Geometry: final body of the model. Coordinates: model frame, mm. A direction names the side the tool comes from. Round coordinates to 2 decimals unless told otherwise and drop trailing zeros. Order: outer loops, then holes, each group sorted by start corner. A loop starts at its lowest first (then second) coordinate and runs counter-clockwise, first axis right, second up. Notation, with made-up numbers: M 65,24.5 L 81,24.5 A17 cw 81,53.5 Z; hole C 30,-39.75 d1. An arc over 180 degrees is marked long. Put each result on its own line as item: value. Start each with the question number.
1) Access query for faces 5 (the cylindrical face through (-12.347, 2.37, -0.275)), 6 (the flat face through (-8, 0, 0)). Directions: +Z, -Z, +X, -X, +Y, -Y. A direction counts if a zero-diameter tool reaches every point of the face in a straight line with its end or side. Return the directions, or none.
2) Draft query along Z for faces 1 (the flat face through (-6, 3.175, 0)), 2 (the flat face through (-6, 2, -1.588)), 3 (the flat face through (-6, 2, 1.588)), 4 (the flat face through (-11, 1.588, 0)). Return one class per face: pulls with the +Z half, pulls with the -Z half, needs draft (parallel to the pull), parting line crosses it, or undercut.
3) Section C-C, the plane y = 2.2. Return loops of the section in (x, z) (1 decimal), then the cut area to 3 significant figures.
4) First-contact query: P1, Ø0.8, axis at x = -11, z = 0, coming from the +Y side; P2, Ø1, axis at x = -11, z = 0, coming from the -Y side. Flat tips, straight axial feed; report the tip coordinate or a pass-through.
5) Section B-B, the plane x = -1.25. Return loops of the section in (y, z) (1 decimal).
6) Material intervals for probe 1 along X at (y, z) = (2.3, 0); probe 2 along X at (y, z) = (1.85, -0.3); probe 3 along X at (y, z) = (1.1, -0.05), sorted ascending. Write a range as [from, to].
from build123d import *

# Parameters (mm, degrees)
BOSS_EXTRUDE2_DEPTH = 3.175
SKETCH1_6_W         = 3.175
SKETCH1_6_H         = 3.175
SKETCH1_6_R         = 1.27
BOSS_EXTRUDE6_DEPTH = 3.175
SKETCH1_8_R         = 1.27
BOSS_EXTRUDE7_DEPTH = 1.5875


with BuildPart() as part:
    # Sketch1 → Boss-Extrude2 (new body)
    with BuildSketch(Plane(origin=(0, 0, 0), x_dir=(1, 0, 0), z_dir=(0, 1, 0))):
        with BuildLine():
            Line((-2.749630657, 1.5875), (-9.525, 1.5875))
            Line((-9.525, 1.5875), (-9.525, -1.5875))
            Line((-9.525, -1.5875), (-2.749630657, -1.5875))
            Line((-2.749630657, -1.5875), (0, -1.5875))
            ThreePointArc((0, -1.5875), (-1.5875, 0), (0, 1.5875))
            Line((0, 1.5875), (-2.749630657, 1.5875))
        make_face()
    extrude(amount=BOSS_EXTRUDE2_DEPTH)

    # Sketch1<6> → Boss-Extrude6 (add)
    with BuildSketch(Plane(origin=(0, 0, 0), x_dir=(1, 0, 0), z_dir=(0, 1, 0))):
        with Locations((-11.1125, 0)):
            Rectangle(SKETCH1_6_W, SKETCH1_6_H)
        with Locations(Location((-11.107619253, 0, 0), (0, 0, 270))):
            Circle(SKETCH1_6_R, mode=Mode.SUBTRACT)
    extrude(amount=BOSS_EXTRUDE6_DEPTH)

    # Sketch1<8> → Boss-Extrude7 (add)
    with BuildSketch(Plane(origin=(0, 0, 0), x_dir=(1, 0, 0), z_dir=(0, 1, 0))):
        with Locations(Location((-11.107619253, 0, 0), (0, 0, 270))):
            Circle(SKETCH1_8_R)
    extrude(amount=BOSS_EXTRUDE7_DEPTH)


solid = part.part
Result sheet:
1. face 5: +Y
1. face 6: +Z, -Z, +X, -X, -Y
2. face 1: needs draft
2. face 2: pulls with the -Z half
2. face 3: pulls with the +Z half
2. face 4: undercut
3. outline: M -12.7,-1.6 L 0,-1.6 A1.6 cw 0,1.6 L -12.7,1.6 Z; hole C -11.1,0 d2.5
3. area: 31.3 mm2
4. P1: stops at y = 1.59
4. P2: stops at y = 0
5. outline: M 0,-1.6 L 3.2,-1.6 L 3.2,-1 L 0,-1 Z; M 0,1 L 3.2,1 L 3.2,1.6 L 0,1.6 Z
6. probe 1: x = [-12.7, -12.38], [-9.84, -1.59]
6. probe 2: x = [-12.7, -12.34], [-9.87, -1.56]
6. probe 3: x = [-12.7, -1.59]
